from build123d import *

# Parameters (mm, degrees)
SKETCH1_R               = 12.5
SKETCH1_R_2             = 5.1
BOSS_EXTRUDE1_DEPTH     = 15
SKETCH2_R               = 41
SKETCH2_R_2             = 5.1
BOSS_EXTRUDE2_DEPTH     = 20
SKETCH3_R               = 3
CUT_EXTRUDE1_DEPTH      = 36
BOSS_EXTRUDE3_DEPTH     = 35
SKETCH5_R               = 1.5
CUT_EXTRUDE2_DEPTH      = 46.2
CUT_EXTRUDE2_DEPTH_BACK = 37.8
SKETCH6_R               = 41
SKETCH6_R_2             = 12.5
CUT_EXTRUDE3_DEPTH      = 10
SKETCH8_R               = 2.5
CUT_EXTRUDE4_DEPTH      = 36.0000001


with BuildPart() as part:
    # Sketch1 → Boss-Extrude1 (new body)
    with BuildSketch(Plane(origin=(0, 0, 0), x_dir=(1, 0, 0), z_dir=(0, 1, 0))):
        Circle(SKETCH1_R)
        Circle(SKETCH1_R_2, mode=Mode.SUBTRACT)
    extrude(amount=BOSS_EXTRUDE1_DEPTH)

    # Sketch2 → Boss-Extrude2 (add)
    with BuildSketch(Plane(origin=(0, 15, 0), x_dir=(1, 0, 0), z_dir=(0, 1, 0))):
        Circle(SKETCH2_R)
        Circle(SKETCH2_R_2, mode=Mode.SUBTRACT)
    extrude(amount=BOSS_EXTRUDE2_DEPTH)

    # Sketch3 → Cut-Extrude1 (cut, through all)
    with BuildSketch(Plane(origin=(0, 35, 0), x_dir=(1, 0, 0), z_dir=(0, 1, 0))):
        with Locations((0, 35)):
            Circle(SKETCH3_R)
        with Locations((30.310889132, 17.5)):
            Circle(SKETCH3_R)
        with Locations((30.310889132, -17.5)):
            Circle(SKETCH3_R)
        with Locations((0, -35)):
            Circle(SKETCH3_R)
        with Locations((-30.310889132, -17.5)):
            Circle(SKETCH3_R)
        with Locations((-30.310889132, 17.5)):
            Circle(SKETCH3_R)
    extrude(amount=-CUT_EXTRUDE1_DEPTH, mode=Mode.SUBTRACT)

    # Sketch4 → Boss-Extrude3 (add)
    with BuildSketch(Plane.XZ):
        with BuildLine():
            ThreePointArc((2.893095228, 4.2), (0, 5.1), (-2.893095228, 4.2))
            Line((-2.893095228, 4.2), (2.893095228, 4.2))
        make_face()
    extrude(amount=-BOSS_EXTRUDE3_DEPTH)

    # Sketch5 → Cut-Extrude2 (cut, two sides)
    with BuildSketch(Plane(origin=(0, 0, 4.2), x_dir=(-1, 0, 0), z_dir=(0, 0, -1))) as cut_extrude2_sk:
        with Locations((0, 9)):
            Circle(SKETCH5_R)
    extrude(amount=CUT_EXTRUDE2_DEPTH, mode=Mode.SUBTRACT)
    extrude(cut_extrude2_sk.sketch, amount=-CUT_EXTRUDE2_DEPTH_BACK, mode=Mode.SUBTRACT)

    # Sketch6 → Cut-Extrude3 (cut)
    with BuildSketch(Plane.XZ.offset(-15)):
        Circle(SKETCH6_R)
        Circle(SKETCH6_R_2, mode=Mode.SUBTRACT)
    extrude(amount=-CUT_EXTRUDE3_DEPTH, mode=Mode.SUBTRACT)

    # Sketch8 → Cut-Extrude4 (cut, through all)
    with BuildSketch(Plane.XZ):
        with Locations((22.5, 0)):
            Circle(SKETCH8_R)
        with Locations((-23.5, 0)):
            Circle(SKETCH8_R)
        with Locations((-11.25, -19.485571585)):
            Circle(SKETCH8_R)
        with Locations((-11.25, 19.485571585)):
            Circle(SKETCH8_R)
        with Locations((11.75, 20.351596989)):
            Circle(SKETCH8_R)
        with Locations((11.75, -20.351596989)):
            Circle(SKETCH8_R)
    extrude(amount=-CUT_EXTRUDE4_DEPTH, mode=Mode.SUBTRACT)


solid = part.part
Can you work these out from the model? Positions are in its coordinate system, mm. A direction names the side the tool comes from. Give positions to 0.01 mm unless a question says otherwise; leave off trailing zeros. Order: outer loops, then holes, each group sorted by start corner. A loop starts at its lowest first (then second) coordinate and runs counter-clockwise, first axis right, second up. Notation, with made-up numbers: M 4.25,84.25 L 20.25,84.25 A16 ccw 20.25,90.25 Z; hole C 88.25,44.25 d4. An arc over 180 degrees is marked long. One line per question, with ' | ' between items.
Item 1: I'm going to push flat-ended pins straight in: pin 1 Ø10 at (x, y) = (-15, 26) entering from -Z; pin 2 Ø6.5 at (x, z) = (11.75, -20.35) entering from -Y; pin 3 Ø12 at (x, y) = (16.5, 9) entering from -Z. Where does each tip first touch, or does it pass through?
Answer block:
pin 1: stops at z = -39.76 | pin 2: stops at y = 25 | pin 3: stops at z = -6.78
Item 2: Suppose I cut it at A-A, the plane x = -23.5. Write out the boundary of the cut face in (y, z), then the cut area to 3 significant figures.
Answer block:
outline: M 25,-33.6 L 35,-33.6 L 35,-2.5 L 25,-2.5 Z; M 25,2.5 L 35,2.5 L 35,33.6 L 25,33.6 Z | area: 622 mm2
Item 3: Suppose I cut it at B-B, the plane z = 0. Write out the boundary of the cut face in (x, y), then the cut area to 3 significant figures.
Answer block:
outline: M -41,25 L -26,25 L -26,35 L -41,35 Z; M -21,25 L -12.5,25 L -12.5,0 L -5.1,0 L -5.1,35 L -21,35 Z; M 5.1,0 L 12.5,0 L 12.5,25 L 20,25 L 20,35 L 5.1,35 Z; M 25,25 L 41,25 L 41,35 L 25,35 Z | area: 988 mm2
Item 4: We'd pull the mould along X, two halves only. Please class faces 1 (the face through (0, 0, 5)), 2 (the face through (-9, 30, 40)), 3 (the face through (-11.575, 29.93, -17.007)): released by +X, released by -X, zero draft, split by the parting line, or undercut.
Answer block:
face 1: zero draft | face 2: split by the parting line | face 3: undercut
Item 5: For faces 4 (the face through (9, 35, -1)), 5 (the face through (0, 17, 4.2)), 6 (the face through (11.923, 12.325, 3.755)), which set-ups out of +Z, -Z, +X, -X, +Y, -Y let a thin tool reach every point of the face, with its end or its side?
Answer block:
face 4: +Z, -Z, +X, -X, +Y | face 5: +Y, -Y | face 6: -Y
Item 6: Please list where these lines run through material, in increasing order: L1, parallel to Z at x = 0, y = 23.5; L2, parallel to X at y = 9, z = 0; L3, parallel to Z at x = -11.25, y = 32.
Answer block:
L1: z = -12.5 to -5.1, 4.2 to 12.5 | L2: x = -12.5 to -5.1, 5.1 to 12.5 | L3: z = -39.43 to -21.99, -16.99 to 16.99, 21.99 to 39.43
Item 7: Suppose I cut it at D-D, the plane z = 35. Write out the boundary of the cut face in (x, y), then the cut area to 3 significant figures.
Answer block:
outline: M -21.35,25 L -3,25 L -3,35 L -21.35,35 Z; M 3,25 L 21.35,25 L 21.35,35 L 3,35 Z | area: 367 mm2
Item 8: Suppose I cut it at C-C, the plane y = 9. Write out the boundary of the cut face in (x, z).
Answer block:
outline: M -2.89,4.2 L -1.5,4.2 L -1.5,12.41 A12.5 ccw -1.5,-12.41 L -1.5,-4.87 A5.1 cw Z; M 1.5,-12.41 A12.5 ccw 1.5,12.41 L 1.5,4.2 L 2.89,4.2 A5.1 cw 1.5,-4.87 Z
